Source: CAD feature listing. Evaluate the final solid. Frame: model axes, mm. Face numbers are marked on the shaded views. A direction names the side the tool comes from. Coordinates: 2 decimals unless noted, no trailing zeros. Write each loop counter-clockwise with the first axis right and the second up, starting at its lowest first coordinate (ties: lowest second). Pieces come first, ordered by that corner, then holes. Notation, with made-up numbers: M 32,26 L 65,26 A3 cw 65,30 Z; hole C 67,-35 d7. An arc over 180 degrees is marked long. One line per item, written item: value. Start each with the question number.
Item 1: Set-up query: the marked faces 5, 6 and 7. Return all of +Z, -Z, +X, -X, +Y, -Y with unobstructed straight access to the full face (end or side cutting, diameter ignored); none if empty.
Item 2: Mould query, pull axis Z, two halves, no side actions, for the marked faces 1, 2, 3 and 4. Classes: released by +Z, released by -Z, zero draft, split by the parting line, or undercut.
Item 3: Cut plane C-C, the plane x = 17.75. Output: boundary loops of the cut face in (y, z), then the cut area to 3 significant figures.
Item 4: Cut plane D-D, the plane y = 2. Output: boundary loops of the cut face in (x, z), then the cut area to 3 significant figures.
Item 5: Ray query, L1, parallel to Y at x = 21.5, z = 1; L2, parallel to Y at x = 6.5, z = 3.5; L3, parallel to X at y = 0.25, z = 3.25. Return the intervals inside material, ascending. Write a range as from..to.
Item 6: Cut plane B-B, the plane z = -0.25. Output: boundary loops of the cut face in (x, y), then the cut area to 3 significant figures.
Item 7: Cut plane A-A, the plane x = 8.25. Output: boundary loops of the cut face in (y, z).
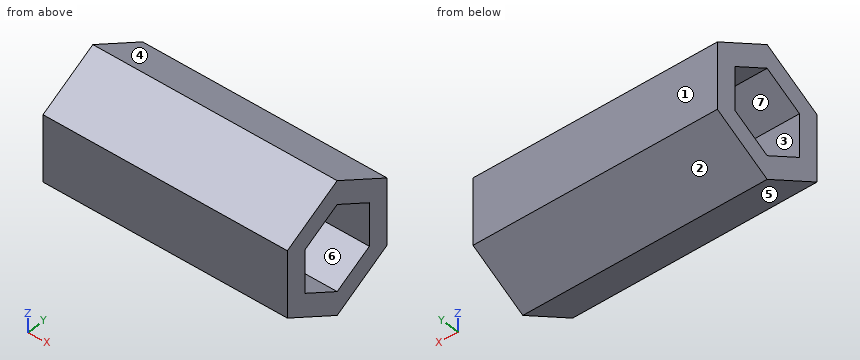
```python
from build123d import *

# Parameters (mm, degrees)
BOSS_EXTRUDE5_DEPTH = 25.4
BOSS_EXTRUDE6_DEPTH = 22.86
CUT_EXTRUDE2_DEPTH  = 10.16
CUT_EXTRUDE4_DEPTH  = 10.16


with BuildPart() as part:
    # Sketch5 → Boss-Extrude5 (new body)
    with BuildSketch(Plane(origin=(0, 0, 0), x_dir=(0, 0, -1), z_dir=(1, 0, 0))):
        Polygon((4, 0), (2, 3.464101615), (-2, 3.464101615), (-4, 0), (-2, -3.464101615), (2, -3.464101615), align=None)
    extrude(amount=BOSS_EXTRUDE5_DEPTH)

    # Sketch7 → Boss-Extrude6 (add)
    with BuildSketch(Plane(origin=(25.4, 0, 0), x_dir=(0, 0, -1), z_dir=(1, 0, 0))):
        Polygon((6.165569463, 0), (3.082784731, 5.339539784), (-3.082784731, 5.339539784), (-6.165569463, 0), (-3.082784731, -5.339539784), (3.082784731, -5.339539784), align=None)
    extrude(amount=-BOSS_EXTRUDE6_DEPTH)

    # Sketch8 → Cut-Extrude2 (cut)
    with BuildSketch(Plane.ZY):
        Polygon((4, 0), (2, 3.464101615), (-2, 3.464101615), (-4, 0), (-2, -3.464101615), (2, -3.464101615), align=None)
    extrude(amount=-CUT_EXTRUDE2_DEPTH, mode=Mode.SUBTRACT)

    # Sketch12 → Cut-Extrude4 (cut)
    with BuildSketch(Plane(origin=(25.4, 0, 0), x_dir=(0, 0, -1), z_dir=(1, 0, 0))):
        Polygon((1.992845787, 3.451710154), (-1.992845787, 3.451710154), (-3.985691573, 0), (-1.992845787, -3.451710154), (1.992845787, -3.451710154), (3.985691573, 0), align=None)
    extrude(amount=-CUT_EXTRUDE4_DEPTH, mode=Mode.SUBTRACT)


solid = part.part
```
From the geometry:
1. face 5: -Z, +X, -X, -Y
1. face 6: +X
1. face 7: -X
2. face 1: zero draft
2. face 2: released by -Z
2. face 3: undercut
2. face 4: released by +Z
3. outline: M -5.34,-3.08 L 0,-6.17 L 5.34,-3.08 L 5.34,3.08 L 0,6.17 L -5.34,3.08 Z; hole M -3.45,-1.99 L 0,-3.99 L 3.45,-1.99 L 3.45,1.99 L 0,3.99 L -3.45,1.99 Z
3. area: 57.5 mm²
4. outline: M 2.54,-5.01 L 25.4,-5.01 L 25.4,-2.83 L 15.24,-2.83 L 15.24,2.83 L 25.4,2.83 L 25.4,5.01 L 2.54,5.01 L 2.54,2.85 L 10.16,2.85 L 10.16,-2.85 L 2.54,-2.85 Z
4. area: 128 mm²
5. L1: y = -5.34..-3.45, 3.45..5.34
5. L2: y = -4.62..-0.87, 0.87..4.62
5. L3: x = 10.16..15.24
6. outline: M 2.54,-5.34 L 25.4,-5.34 L 25.4,-3.45 L 15.24,-3.45 L 15.24,3.45 L 25.4,3.45 L 25.4,5.34 L 2.54,5.34 L 2.54,3.46 L 10.16,3.46 L 10.16,-3.46 L 2.54,-3.46 Z
6. area: 121 mm²
7. outline: M -5.34,-3.08 L 0,-6.17 L 5.34,-3.08 L 5.34,3.08 L 0,6.17 L -5.34,3.08 Z; hole M -3.46,-2 L 0,-4 L 3.46,-2 L 3.46,2 L 0,4 L -3.46,2 Z
